Read the model definition and answer for the solid it produces. Units are mm, in the model's axes. A direction names the side the tool comes from. Round coordinates to 2 decimals unless told otherwise and drop trailing zeros. Write each loop counter-clockwise with the first axis right and the second up, starting at its lowest first coordinate (ties: lowest second). Pieces come first, ordered by that corner, then holes.
from build123d import *

# Parameters (mm, degrees)
SKETCH1_W           = 27
SKETCH1_H           = 5
BOSS_EXTRUDE1_DEPTH = 3
SKETCH2_R           = 2.5
BOSS_EXTRUDE2_DEPTH = 8
SKETCH3_R           = 2.5
BOSS_EXTRUDE3_DEPTH = 7


with BuildPart() as part:
    # Sketch1 → Boss-Extrude1 (new body)
    with BuildSketch(Plane(origin=(0, 0, 0), x_dir=(0, 0, -1), z_dir=(1, 0, 0))):
        Rectangle(SKETCH1_W, SKETCH1_H)
    extrude(amount=BOSS_EXTRUDE1_DEPTH)

    # Sketch2 → Boss-Extrude2 (add)
    with BuildSketch(Plane(origin=(3, 0, 0), x_dir=(0, 0, -1), z_dir=(1, 0, 0))):
        with Locations((-13.5, 0)):
            Circle(SKETCH2_R)
    extrude(amount=-BOSS_EXTRUDE2_DEPTH)

    # Sketch3 → Boss-Extrude3 (add)
    with BuildSketch(Plane.ZY):
        with Locations((-13.5, 0)):
            Circle(SKETCH3_R)
    extrude(amount=-BOSS_EXTRUDE3_DEPTH)


solid = part.part
Q1. Section A-A (y = 2) is taken. Determine the outline of the cut face in (x, z).
Verdict:
outline: (-5, 12) - (0, 12) - (0, -15) - (7, -15) - (7, -12) - (3, -12) - (3, 15) - (-5, 15) - close
Q2. Section B-B (z = 0) is taken. Determine the outline of the cut face in (x, y).
Verdict:
outline: (0, -2.5) - (3, -2.5) - (3, 2.5) - (0, 2.5) - close
Q3. Which of the six approach directions +Z, -Z, +X, -X, +Y, -Y give full straight-line access (tool end or side, diameter ignored) to faces 1 (the cylindrical face through (4, 0, -16)), 2 (the cylindrical face through (-2, 0, 16)), 3 (the flat face through (1, 2.5, 0))?
Verdict:
face 1: +X
face 2: -X
face 3: +Z, -Z, +X, -X, +Y
Q4. Section C-C (x = 5) is taken. Determine the outline of the cut face in (y, z), then the cut area to 3 significant figures.
Verdict:
outline: circle Ø5 at (0, -13.5)
area: 19.6 mm2
Q5. Section D-D (y = -0.8) is taken. Determine the outline of the cut face in (x, z).
Verdict:
outline: (-5, 11.13) - (0, 11.13) - (0, -15.87) - (7, -15.87) - (7, -11.13) - (3, -11.13) - (3, 15.87) - (-5, 15.87) - close
Q6. Straight lines are drawn through the part: probe 1 along X at (y, z) = (-0.25, -12.5); probe 2 along X at (y, z) = (0.6, -4); probe 3 along Z at (x, y) = (5, -1.5). For each, find the intervals that lie inside material, in ascending order.
Verdict:
probe 1: x = 0 to 7
probe 2: x = 0 to 3
probe 3: z = -15.5 to -11.5
Q7. Flat-ended cylindrical pins translate along their axes: pin 1 Ø5 at (x, z) = (5, -1.5) entering from -Y; pin 2 Ø2 at (y, z) = (-0.5, -11) entering from -X; pin 3 Ø5 at (x, z) = (-3, 7) entering from -Y. Find the tip coordinate at first contact, or state that the pin passes through.
Verdict:
pin 1: stops at y = -2.5
pin 2: stops at x = 0
pin 3: passes through
